from build123d import *

# Parameters (mm, degrees)
SKETCH1_R           = 2.5
SKETCH1_W           = 3
SKETCH1_H           = 25
BOSS_EXTRUDE1_DEPTH = 3


with BuildPart() as part:
    # Sketch1 → Boss-Extrude1 (new body)
    with BuildSketch(Plane(origin=(0, 0, 0), x_dir=(1, 0, 0), z_dir=(0, 1, 0))):
        Polygon((-29.5, 32.5), (-29.5, 12.5), (-29.5, -12.5), (-29.5, -32.5), (29.5, -32.5), (29.5, -12.5), (29.5, 12.5), (29.5, 32.5), align=None)
        with Locations((-22.980970389, -22.980970389)):
            Circle(SKETCH1_R, mode=Mode.SUBTRACT)
        with Locations((22.980970389, -22.980970389)):
            Circle(SKETCH1_R, mode=Mode.SUBTRACT)
        with Locations((-15, 0)):
            Rectangle(SKETCH1_W, SKETCH1_H, mode=Mode.SUBTRACT)
        with Locations((-22.980970389, 22.980970389)):
            Circle(SKETCH1_R, mode=Mode.SUBTRACT)
        with Locations((15, 0)):
            Rectangle(SKETCH1_W, SKETCH1_H, mode=Mode.SUBTRACT)
        with Locations((22.980970389, 22.980970389)):
            Circle(SKETCH1_R, mode=Mode.SUBTRACT)
    extrude(amount=BOSS_EXTRUDE1_DEPTH)


solid = part.part
Can you work these out from the model? Positions are in its coordinate system, mm. A direction names the side the tool comes from. Coordinates: 2 decimals unless noted, no trailing zeros. Order: outer loops, then holes, each group sorted by start corner. A loop starts at its lowest first (then second) coordinate and runs counter-clockwise, first axis right, second up. Notation, with made-up numbers: M -27.5,61.25 L 8.5,61.25 A21 cw 8.5,78.25 Z; hole C 42,48 d8. An arc over 180 degrees is marked long. Write item = value, one per line.
(1) I need wall thicknesses on line 1 along X through (y, z) = (2.7, 9); line 2 along Z through (x, y) = (-14.5, 1.15); line 3 along X through (y, z) = (1.1, -23.5). Which ranges of each line are inside material? Lowest first, please. Write a range as [from, to].
Results are:
line_1 = [-29.5, -16.5], [-13.5, 13.5], [16.5, 29.5]
line_2 = [-32.5, -12.5], [12.5, 32.5]
line_3 = [-29.5, -25.43], [-20.54, 20.54], [25.43, 29.5]
(2) Suppose I cut it at B-B on y = 0.6. Please give me the cut outline in (x, z), plus the area to 3 significant figures.
Results are:
outline = M -29.5,-32.5 L 29.5,-32.5 L 29.5,32.5 L -29.5,32.5 Z; hole C -22.98,-22.98 d5; hole C -22.98,22.98 d5; hole M -16.5,-12.5 L -13.5,-12.5 L -13.5,12.5 L -16.5,12.5 Z; hole M 13.5,-12.5 L 16.5,-12.5 L 16.5,12.5 L 13.5,12.5 Z; hole C 22.98,-22.98 d5; hole C 22.98,22.98 d5
area = 3,610 mm2
(3) Suppose I cut it at C-C on x = -24.5. Please give me the cut outline in (y, z).
Results are:
outline = M 0,-32.5 L 3,-32.5 L 3,-24.97 L 0,-24.97 Z; M 0,-21 L 3,-21 L 3,21 L 0,21 Z; M 0,24.97 L 3,24.97 L 3,32.5 L 0,32.5 Z
(4) For faces 1 (the face through (0, 1, -32.5)), 2 (the face through (-15, 1, -12.5)), which set-ups out of +Z, -Z, +X, -X, +Y, -Y let a thin tool reach every point of the face, with its end or its side?
Results are:
face_1 = -Z, +X, -X, +Y, -Y
face_2 = +Y, -Y
(5) Suppose I cut it at A-A on z = 9.5. Please give me the cut outline in (x, y), plus the area to 3 significant figures.
Results are:
outline = M -29.5,0 L -16.5,0 L -16.5,3 L -29.5,3 Z; M -13.5,0 L 13.5,0 L 13.5,3 L -13.5,3 Z; M 16.5,0 L 29.5,0 L 29.5,3 L 16.5,3 Z
area = 159 mm2
